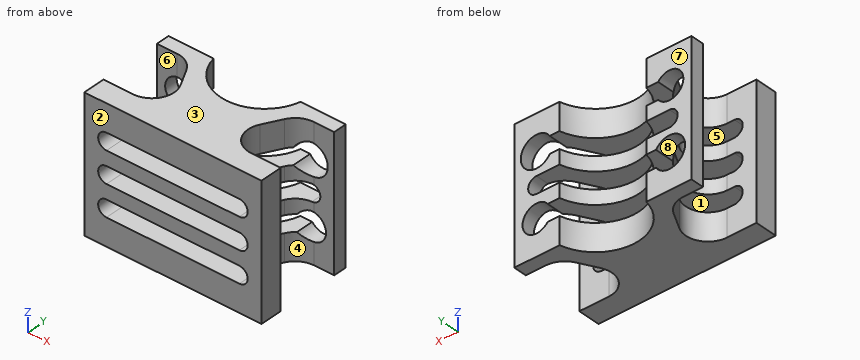
```python
from build123d import *

# Parameters (mm, degrees)
BOSS_EXTRUDE1_DEPTH     = 38.1
CUT_EXTRUDE2_DEPTH      = 71.436357089
FILLET1_R               = 6.35
SKETCH4_W               = 50.8
SKETCH4_H               = 2.54
CUT_EXTRUDE3_DEPTH      = 71.436357187
CUT_EXTRUDE5_DEPTH      = 5.08
CUT_EXTRUDE5_DEPTH_BACK = 25.4
SKETCH5_R               = 4.5
SKETCH5_R_2             = 4


with BuildPart() as part:
    # Sketch1 → Boss-Extrude1 (new body)
    with BuildSketch(Plane.XY):
        with BuildLine():
            Line((38.1, 30.48), (50.8, 30.48))
            Line((50.8, 30.48), (50.8, 24.13))
            Line((50.8, 24.13), (41.275, 24.13))
            Line((41.275, 24.13), (31.75, 6.35))
            Line((31.75, 6.35), (50.8, 6.35))
            Line((50.8, 6.35), (50.8, 0))
            Line((50.8, 0), (0, 0))
            Line((0, 0), (0, 6.35))
            Line((0, 6.35), (19.05, 6.35))
            Line((19.05, 6.35), (9.525, 24.13))
            Line((9.525, 24.13), (0, 24.13))
            Line((0, 24.13), (0, 30.48))
            Line((0, 30.48), (12.7, 30.48))
            ThreePointArc((12.7, 30.48), (25.4, 17.78), (38.1, 30.48))
        make_face()
    extrude(amount=BOSS_EXTRUDE1_DEPTH)

    # Sketch3 → Cut-Extrude2 (cut, through all)
    with BuildSketch(Plane.XZ):
        with BuildLine():
            Line((6.35, 21.43125), (44.45, 21.43125))
            ThreePointArc((44.45, 21.43125), (46.83125, 19.05), (44.45, 16.66875))
            Line((44.45, 16.66875), (6.35, 16.66875))
            ThreePointArc((6.35, 16.66875), (3.96875, 19.05), (6.35, 21.43125))
        make_face()
        with BuildLine():
            Line((6.35, 30.32125), (44.45, 30.32125))
            ThreePointArc((44.45, 30.32125), (46.83125, 27.94), (44.45, 25.55875))
            Line((44.45, 25.55875), (6.35, 25.55875))
            ThreePointArc((6.35, 25.55875), (3.96875, 27.94), (6.35, 30.32125))
        make_face()
        with BuildLine():
            Line((6.35, 12.54125), (44.45, 12.54125))
            ThreePointArc((44.45, 12.54125), (46.83125, 10.16), (44.45, 7.77875))
            Line((44.45, 7.77875), (6.35, 7.77875))
            ThreePointArc((6.35, 7.77875), (3.96875, 10.16), (6.35, 12.54125))
        make_face()
    extrude(amount=-CUT_EXTRUDE2_DEPTH, mode=Mode.SUBTRACT)

    # Fillet1
    fillet1_edges = [part.edges().sort_by_distance(p)[0] for p in [
        (41.275, 24.13, 3.889375),
        (41.275, 24.13, 34.210625),
        (19.05, 6.35, 34.210625),
        (19.05, 6.35, 23.495),
        (19.05, 6.35, 14.605),
        (19.05, 6.35, 3.889375),
        (31.75, 6.35, 34.210625),
        (31.75, 6.35, 23.495),
        (31.75, 6.35, 14.605),
        (31.75, 6.35, 3.889375),
        (9.525, 24.13, 34.210625),
        (9.525, 24.13, 23.495),
        (9.525, 24.13, 14.605),
        (9.525, 24.13, 3.889375),
        (41.275, 24.13, 23.495),
        (41.275, 24.13, 14.605),
    ]]
    fillet(fillet1_edges, radius=FILLET1_R)

    # Sketch4 → Cut-Extrude3 (cut, through all)
    with BuildSketch(Plane.XY.offset(38.1)):
        with Locations((25.4, 29.21)):
            Rectangle(SKETCH4_W, SKETCH4_H)
    extrude(amount=-CUT_EXTRUDE3_DEPTH, mode=Mode.SUBTRACT)

    # Sketch5 → Cut-Extrude5 (cut, two sides: drawn at the far end of the back side and taken through both)
    with BuildSketch(Plane.XZ.offset(-24.13).offset(-CUT_EXTRUDE5_DEPTH_BACK)):
        with Locations((44.45, 27.94)):
            Circle(SKETCH5_R)
        with Locations((6.35, 27.94)):
            Circle(SKETCH5_R_2)
        with Locations((6.35, 10.16)):
            Circle(SKETCH5_R)
        with Locations((44.45, 10.16)):
            Circle(SKETCH5_R_2)
    extrude(amount=CUT_EXTRUDE5_DEPTH + CUT_EXTRUDE5_DEPTH_BACK, mode=Mode.SUBTRACT)


solid = part.part
```
Work out the finished part from the listing and answer in its coordinate system (mm). Face numbers are marked on the shaded views. A direction names the side the tool comes from. Round coordinates to 2 decimals unless told otherwise and drop trailing zeros. Loops run counter-clockwise (first coordinate to the right, second up) from the corner with the lowest first, then second, coordinate; pieces in that order, holes last. Notation, with made-up numbers: M 63.5,2.5 L 90.5,2.5 A29 ccw 90.5,41.5 Z; hole C -33,76.5 d1. An arc over 180 degrees is marked long. One line per question, with ' | ' between items.
Q1. This flat-tipped pin is pushed along its axis until it touches: pin 1 Ø7 at (x, z) = (6.35, 27.94) entering from +Y. Where does it stop, or does it pass through?
Conclusion:
pin 1: stops at y = 6.37
Q2. The mould has two halves that part along Z. Classify the marked faces 1, 2 and 3: +Z half, -Z half, draft (parallel to the pull), parting line (faces both ways), or undercut.
Conclusion:
face 1: undercut | face 2: draft | face 3: +Z half
Q3. Find section B-B, the plane y = 21.75. State how many separate pieces and enclosed holes the cut face has, then the cut area to 3 significant figures.
Conclusion:
separate pieces: 8 | enclosed holes: 0 | area: 262 mm2
Q4. A tool of negligible diameter and unlimited length cuts with its end or side. For the marked faces 4, 5, 6, 7 and 8, from which of +Z, -Z, +X, -X, +Y, -Y can it reach the whole face along a straight path? Write none if from no direction.
Conclusion:
face 4: +Z, -Z, +X | face 5: +Y, -Y | face 6: +Z, -Z, -X | face 7: +Z, -Z, +X, -X, +Y | face 8: +Y
Q5. Consider line 1 along Z through (x, y) = (44.45, 24.5); line 2 along Z through (x, y) = (23, 5.5); line 3 along X through (y, z) = (26, 27.94). Determine where each line is inside the solid, lowest interval first. Write a range as from..to.
Conclusion:
line 1: z = 0..6.16, 14.16..16.67, 21.43..23.44, 32.44..38.1 | line 2: z = 0..7.78, 12.54..16.67, 21.43..25.56, 30.32..38.1 | line 3: x = 0..2.35, 48.95..50.8
Q6. Find section D-D, the plane x = 19. Give the vertices of the cut face in (y, z), then the cut area to 3 significant figures.
Conclusion:
outline: M 0,0 L 19.51,0 L 19.51,7.78 L 0,7.78 Z; M 0,12.54 L 19.51,12.54 L 19.51,16.67 L 0,16.67 Z; M 0,21.43 L 19.51,21.43 L 19.51,25.56 L 0,25.56 Z; M 0,30.32 L 19.51,30.32 L 19.51,38.1 L 0,38.1 Z | area: 465 mm2
Q7. Find section A-A, the plane z = 19.05. Give the vertices of the cut face in (x, y), then the cut area to 3 significant figures.
Conclusion:
outline: M 0,0 L 3.97,0 L 3.97,6.35 L 0,6.35 Z; M 0,24.13 L 3.97,24.13 L 3.97,27.94 L 0,27.94 Z; M 46.83,0 L 50.8,0 L 50.8,6.35 L 46.83,6.35 Z; M 46.83,24.13 L 50.8,24.13 L 50.8,27.94 L 46.83,27.94 Z | area: 80.6 mm2
